Autodesk Inventor part; units mm, degrees
ref_plane "YZ Plane" through (0, 0, 0) normal (1, 0, 0) x (0, 1, 0)
ref_plane "XZ Plane" through (0, 0, 0) normal (0, 1, 0) x (-1, 0, 0)
ref_plane "XY Plane" through (0, 0, 0) normal (0, 0, 1) x (1, 0, 0)
sketch "Sketch1" plane through (0, 0, 0) normal (0, 1, 0) x (-1, 0, 0)
  line L0 (0, 0) -> (-20.32, 0)
  line L1 (-20.32, 0) -> (-20.32, 79.6462)
  line L2 (-20.32, 79.6462) -> (-13.0825, 94.4853)
  line L3 (133.35, -57.15) -> (0, -57.15)
  line L4 (0, -57.15) -> (0, 0)
  line L5 (25.4, -46.99) -> (69.85, -46.99) construction
  line L6 (107.0012, -42.6627) -> (5.5464, 62.3969) construction
  line L7 (-11.43, 57.15) -> (-11.43, 6.35) construction
  line L8 (164.084, 0) -> (-51.054, 0) construction
  line L9 (133.35, -57.15) -> (-13.0825, 94.4853)
  line L10 (107.0012, -42.6627) -> (113.3962, -36.4872) construction
  point P0 (56.2738, 9.8671)
  dimension "d25" = 50.8
  dimension "d26" = 146.05
  dimension "d27" = 73.025
  dimension "d28" = 44.45
  dimension "d32" = 57.15
  dimension "d33" = 133.35
  dimension "d44" = 20.32
  dimension "d46" = 8.89
  dimension "d47" = 10.16
  dimension "d49" = 25.4
  dimension "d60" = 46
  dimension "d61" = 8.89
  dimension "d64" = 6.35
  dimension "d66" = 28.7247
  dimension "d71" = 70
  dimension "d72" = 16.51
extrude "Plate1" add sketch "Sketch1" along normal blind 1.5875
hole "Hole1" at (-5.5464, 0, 62.3969) at (11.43, 0, 57.15) at (-56.2738, 0, 9.8671) at (-107.0012, 0, -42.6627) at (-69.85, 0, -46.99) at (-25.4, 0, -46.99) at (11.43, 0, 6.35) direction (0, 1, 0) diameter 3.4544 end through all
chamfer "Corner Chamfer1" distance 8.89 angle 45 1 edges at (-133.35, 0.7937, -57.15)
fillet "Corner Round1" radius 6.35 2 edges at (20.32, 0.7937, 0) (0, 0.7937, -57.15)
fillet "Corner Round1" radius 2.54 3 edges at (13.0825, 0.7937, 94.4853) (-127.1745, 0.7937, -50.7551) (-124.46, 0.7937, -57.15)
fillet "Corner Round1" radius 1.27 1 edges at (0, 0.7937, 0)
fillet "Corner Round1" radius 25.4 1 edges at (20.32, 0.7937, 79.6462)
equation "\"BendReliefWidth\" = Thickness"
equation "\"BendReliefDepth\" = 0.5 * Thickness"
equation "\"MinimumRemnant\" = 2 * Thickness"
equation "\"GapSize\" = Thickness"
properties part number "J009838" material "Polycarbonate, Clear"
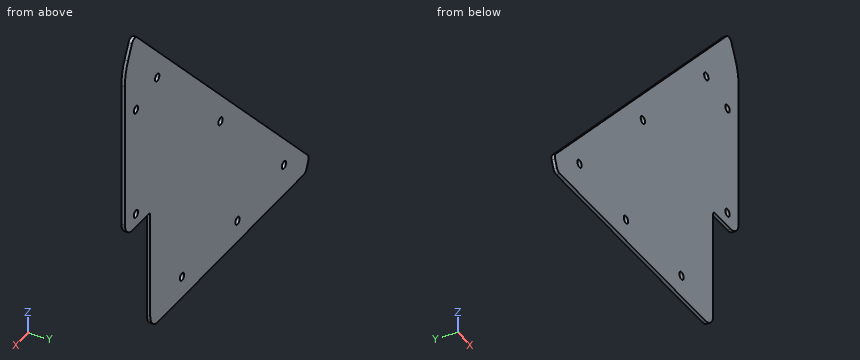
Model file for the job. Use its own axes, mm. Coordinates: 2 decimals unless noted, no trailing zeros. Loops run counter-clockwise (first coordinate to the right, second up) from the corner with the lowest first, then second, coordinate; pieces in that order, holes last. Notation, with made-up numbers: M -32.75,-24.5 L -20.75,-24.5 A12 ccw -20.75,-16.5 Z; hole C -22.5,3.5 d1. An arc over 180 degrees is marked long. Use CSV: the item, a comma, the result in double quotes. Start each with the question number.
1. Band-saw the part on C-C, the plane y = 0.4. List the corners of the cut face in (x, z), then the cut area to 3 significant figures.
2. Band-saw the part on D-D, the plane x = -69.85. List the corners of the cut face in (y, z).
3. Band-saw the part on A-A, the plane z = -46.99. List the corners of the cut face in (x, y).
4. Flat gauge pins, fed straight in: pin 1 (4 mm diameter, centred on x = -5.55, z = 62.4, fed in from +Y); pin 2 (0.8 mm diameter, centred on y = 0.5, z = -32, fed in from +X). Where does each tip first touch, or does it go through?
5. Band-saw the part on B-B, the plane x = -25.4. List the corners of the cut face in (y, z).
6. Probe probe 1 along X at (y, z) = (0.75, -46.99); probe 2 along Z at (x, y) = (11.5, 0.7); probe 3 along Z at (x, y) = (-105.5, 1.4). List the from-to ranges inside material, lowest first. Write a range as [from, to].
Entries:
1,outline,"M -126.52,-52.3 L -125.12,-55.6 A2.54 ccw -122.78,-57.15 L -6.35,-57.15 A6.35 ccw 0,-50.8 L 0,-1.27 A1.27 cw 1.27,0 L 13.97,0 A6.35 ccw 20.32,6.35 L 20.32,73.78 A25.4 ccw 17.75,84.92 L 14.67,91.22 A2.54 ccw 10.56,91.88 L -126.01,-49.55 A2.54 ccw Z; hole C -107,-42.66 d3.45; hole C -69.85,-46.99 d3.45; hole C -56.27,9.87 d3.45; hole C -25.4,-46.99 d3.45; hole C -5.55,62.4 d3.45; hole C 11.43,6.35 d3.45; hole C 11.43,57.15 d3.45"
1,area,"10,900 mm2"
2,outline,"M 0,-57.15 L 1.59,-57.15 L 1.59,-48.72 L 0,-48.72 Z; M 0,-45.26 L 1.59,-45.26 L 1.59,8.61 L 0,8.61 Z"
3,outline,"M -123.54,0 L -71.58,0 L -71.58,1.59 L -123.54,1.59 Z; M -68.12,0 L -27.13,0 L -27.13,1.59 L -68.12,1.59 Z; M -23.67,0 L 0,0 L 0,1.59 L -23.67,1.59 Z"
4,pin 1,"stops at y = 1.59"
4,pin 2,"stops at x = 0"
5,outline,"M 0,-57.15 L 1.59,-57.15 L 1.59,-48.72 L 0,-48.72 Z; M 0,-45.26 L 1.59,-45.26 L 1.59,54.64 L 0,54.64 Z"
6,probe 1,"x = [-123.54, -71.58], [-68.12, -27.13], [-23.67, 0]"
6,probe 2,"z = [0, 4.62], [8.08, 55.42], [58.88, 92.49]"
6,probe 3,"z = [-57.15, -43.52], [-41.81, -28.31]"
